```python
from build123d import *

# Parameters (mm, degrees)
CROQUIS1_W              = 350
CROQUIS1_H              = 40
SALIENTE_EXTRUIR1_DEPTH = 30
CROQUIS2_W              = 24
CROQUIS2_H              = 34
CORTAR_EXTRUIR1_DEPTH   = 890


with BuildPart() as part:
    # Croquis1 → Saliente-Extruir1 (new body)
    with BuildSketch(Plane(origin=(0, 0, 0), x_dir=(0, 0, -1), z_dir=(1, 0, 0))):
        Rectangle(CROQUIS1_W, CROQUIS1_H)
    extrude(amount=SALIENTE_EXTRUIR1_DEPTH)

    # Croquis2 → Cortar-Extruir1 (cut)
    with BuildSketch(Plane.XY.offset(175)):
        with Locations((15, 0)):
            Rectangle(CROQUIS2_W, CROQUIS2_H)
    extrude(amount=-CORTAR_EXTRUIR1_DEPTH, mode=Mode.SUBTRACT)


solid = part.part
```
Check sheet for the modelled part. Datum: model origin and axes. Units: mm. A direction names the side the tool comes from. Round coordinates to 2 decimals unless told otherwise and drop trailing zeros. Order: outer loops, then holes, each group sorted by start corner. A loop starts at its lowest first (then second) coordinate and runs counter-clockwise, first axis right, second up.
1) Scan lines: line 1 (X direction, y = 11.5, z = 100); line 2 (Y direction, x = 7, z = 23.5). Record each from-to range of solid material in increasing order.
2) Section check A-A (y = -8). Record the boundary of the cut face in (x, z).
3) Mould release check, pull along X, two halves, no side actions. Record for faces 3 (the flat face through (30, 0, 2)), 4 (the flat face through (15, -17, 2)), 5 (the flat face through (0, 0, 2)), 6 (the flat face through (1, 0, 175)): +X half, -X half, draft (parallel to the pull), parting line (faces both ways), or undercut.
4) Tool access check on faces 1 (the flat face through (15, 20, 2)), 2 (the flat face through (27, 0, 2)). Record the directions out of +Z, -Z, +X, -X, +Y, -Y that give a thin tool (end or side, any length) a straight path to the whole face; none if there is none.
5) Section check B-B (z = 98). Record the boundary of the cut face in (x, y).
6) Section check C-C (x = 15.25). Record the boundary of the cut face in (y, z).
7) Go/stop test with a flat-tipped pin: pin 1 Ø4 at (y, z) = (-8, -106.5) entering from -X. Record where the tip stops, or that it passes through.
Result:
1. line 1: x = 0 to 3, 27 to 30
1. line 2: y = -20 to -17, 17 to 20
2. outline: (0, -175) - (3, -175) - (3, 175) - (0, 175) - close; (27, -175) - (30, -175) - (30, 175) - (27, 175) - close
3. face 3: +X half
3. face 4: undercut
3. face 5: -X half
3. face 6: draft
4. face 1: +Z, -Z, +X, -X, +Y
4. face 2: +Z, -Z
5. outline: (0, -20) - (30, -20) - (30, 20) - (0, 20) - close; hole (3, -17) - (27, -17) - (27, 17) - (3, 17) - close
6. outline: (-20, -175) - (-17, -175) - (-17, 175) - (-20, 175) - close; (17, -175) - (20, -175) - (20, 175) - (17, 175) - close
7. pin 1: stops at x = 0
